```python
from build123d import *

# Parameters (mm, degrees)
SKETCH1_W           = 40
SKETCH1_H           = 40
BOSS_EXTRUDE1_DEPTH = 15
SKETCH2_R           = 20
BOSS_EXTRUDE2_DEPTH = 20
SKETCH3_W           = 40
SKETCH3_H           = 40
BOSS_EXTRUDE3_DEPTH = 15


with BuildPart() as part:
    # Sketch1 → Boss-Extrude1 (new body)
    with BuildSketch(Plane(origin=(0, 0, 0), x_dir=(1, 0, 0), z_dir=(0, 1, 0))):
        Rectangle(SKETCH1_W, SKETCH1_H)
    extrude(amount=BOSS_EXTRUDE1_DEPTH)

    # Sketch2 → Boss-Extrude2 (add)
    with BuildSketch(Plane(origin=(0, 15, 0), x_dir=(1, 0, 0), z_dir=(0, 1, 0))):
        with Locations(Location((0, 0, 0), (0, 0, 270))):
            Circle(SKETCH2_R)
    extrude(amount=BOSS_EXTRUDE2_DEPTH)

    # Sketch3 → Boss-Extrude3 (add)
    with BuildSketch(Plane(origin=(0, 35, 0), x_dir=(1, 0, 0), z_dir=(0, 1, 0))):
        Rectangle(SKETCH3_W, SKETCH3_H)
    extrude(amount=BOSS_EXTRUDE3_DEPTH)


solid = part.part
```
Could you check a few things on this model? Use its own coordinates, in mm. A direction names the side the tool comes from. Coordinates: 2 decimals unless noted, no trailing zeros. Loops run counter-clockwise (first coordinate to the right, second up) from the corner with the lowest first, then second, coordinate; pieces in that order, holes last.
1) Will this pin go through, and if not, where does the flat tip stop? pin 1 Ø4 at (y, z) = (18.5, -7) entering from -X.
Reported:
pin 1: stops at x = -19.36
2) Imagine slicing it at A-A (x = 16). List the corners of the cut face in (y, z) for me.
Reported:
outline: (0, -20) - (15, -20) - (15, -12) - (35, -12) - (35, -20) - (50, -20) - (50, 20) - (35, 20) - (35, 12) - (15, 12) - (15, 20) - (0, 20) - close
3) Thinking about a two-plate mould opening in Y: for faces 5 (the face through (20, 7, 0)), 6 (the face through (15, 35, -16)), 7 (the face through (0, 0, 0)), 8 (the face through (16, 15, 16)), which applies, released by +Y, released by -Y, zero draft, split by the parting line, or undercut?
Reported:
face 5: zero draft
face 6: undercut
face 7: released by -Y
face 8: undercut
4) Which directions (+Z, -Z, +X, -X, +Y, -Y) give clear straight access to the entire face, cutting with the end or side of a thin tool? Please do faces 1 (the face through (15, 15, -16)), 2 (the face through (-16, 15, 15)), 3 (the face through (-16, 15, -15)), 4 (the face through (-19.524, 24.86, -4.336)).
Reported:
face 1: -Z, +X
face 2: +Z, -X
face 3: -Z, -X
face 4: none
5) Imagine slicing it at C-C (y = 28.5). List the corners of the cut face in (x, z) for me.
Reported:
outline: circle Ø40 at (0, 0)
6) Imagine slicing it at B-B (z = 15). List the corners of the cut face in (x, y) for me, and give its area (3 significant figures).
Reported:
outline: (-20, 0) - (20, 0) - (20, 15) - (13.23, 15) - (13.23, 35) - (20, 35) - (20, 50) - (-20, 50) - (-20, 35) - (-13.23, 35) - (-13.23, 15) - (-20, 15) - close
area: 1,730 mm2
7) Please list where these lines run through material, in increasing order: line 1 along Y through (x, z) = (-18, 14); line 2 along X through (y, z) = (22.5, -5); line 3 along Z through (x, y) = (4, 15.5).
Reported:
line 1: y = 0 to 15, 35 to 50
line 2: x = -19.36 to 19.36
line 3: z = -19.6 to 19.6
